```python
from build123d import *

# Parameters (mm, degrees)
F0_R             = 8
F1_DEPTH         = 1.5
F2_R             = 5.5
F3_DEPTH         = 22.5
F4_R             = 4
F5_DEPTH         = 21.5
F7_D             = 1.7
F9_D             = 3
F11_DEPTH        = 8.001
F11_DEPTH_BACK   = 25
F13_DEPTH        = 4
F13_COPIES_COUNT = 3


# Not quite as in the source:
# - a pattern or mirror of a feature is missing from the dataset's text; its kind, count and spacing are read off the source's solid


with BuildPart() as f1:
    # F0 (on Right) → F1 (new body)
    with BuildSketch(Plane.YZ):
        Circle(F0_R)
    extrude(amount=F1_DEPTH)

    # F2 (on face) → F3 (join)
    with BuildSketch(Plane.YZ.offset(1.5)):
        Circle(F2_R)
    extrude(amount=F3_DEPTH)

    # F4 (on face) → F5 (cut)
    with BuildSketch(Plane.YZ.offset(24)):
        Circle(F4_R)
    extrude(amount=-F5_DEPTH, mode=Mode.SUBTRACT)

    # F7 (through all)
    with Locations(Plane(origin=(0, 0, 0), x_dir=(0, 1, 0), z_dir=(-1, 0, 0))):
        with Locations((-3.25, -5.6291651246), (6.5, 0), (-3.25, 5.6291651246)):
            Hole(F7_D / 2)

    # F9 (through all)
    with Locations(Plane.YZ.offset(2.5)):
        with Locations((0, 0)):
            Hole(F9_D / 2)

    # F10 (on Front) → F11 (cut, two sides)
    with BuildSketch(Plane.XZ) as f11_sk:
        with BuildLine():
            Line((8, -1.75), (19.25, -1.75))
            ThreePointArc((19.25, -1.75), (21, 0), (19.25, 1.75))
            Line((19.25, 1.75), (8, 1.75))
            ThreePointArc((8, 1.75), (6.25, 0), (8, -1.75))
        make_face()
    extrude(amount=-F11_DEPTH, mode=Mode.SUBTRACT)
    extrude(f11_sk.sketch, amount=F11_DEPTH_BACK, mode=Mode.SUBTRACT)

    # F12 (on face) → F13 (cut)
    with BuildSketch(Plane.YZ.offset(1.5)):
        with BuildLine():
            Line((-0.5156865167, -5.4757709427), (-4.4843134833, -3.1844830952))
            ThreePointArc((-4.4843134833, -3.1844830952), (-3.702278018, -4.0673255927), (-2.7500001403, -4.7631396398))
            ThreePointArc((-2.7500001403, -4.7631396398), (-1.6712684341, -5.2399295626), (-0.5156865167, -5.4757709427))
        make_face()
    f13 = extrude(amount=F13_DEPTH, mode=Mode.SUBTRACT)

    # F13_copies: F13 ×3 about axis
    f13_copies_axis = Axis((0, 0, 0), (1, 0, 0))
    for i in range(1, F13_COPIES_COUNT):
        add(f13.rotate(f13_copies_axis, i * 360 / F13_COPIES_COUNT), mode=Mode.SUBTRACT)


solid = f1.part
```
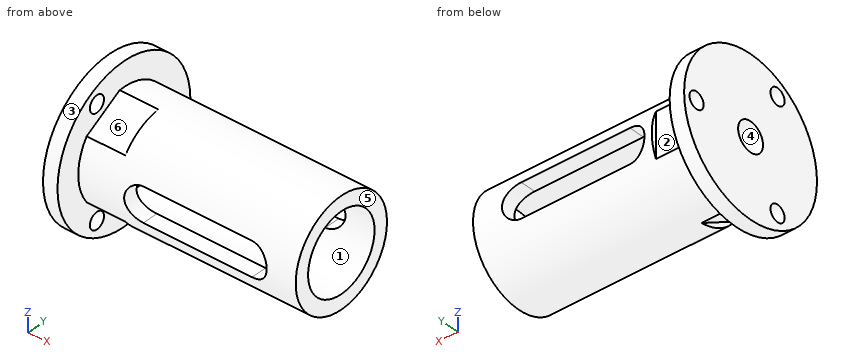
Design review of the part built by this model. Coordinates are the model's own, in mm. Face numbers are marked on the shaded views. A direction names the side the tool comes from. Give positions to 0.01 mm unless a question says otherwise; leave off trailing zeros. Loops run counter-clockwise (first coordinate to the right, second up) from the corner with the lowest first, then second, coordinate; pieces in that order, holes last. Notation, with made-up numbers: M 77.5,4.25 L 102.5,4.25 A17 cw 102.5,19.25 Z; hole C -13,-37.5 d11. An arc over 180 degrees is marked long. Return JSON: item names as keys, results as strings. Group by question number.
Item 1: For probe 1 along X at (y, z) = (-2.5, -4.5); probe 2 along Z at (x, y) = (10, 0); probe 3 along Z at (x, y) = (1.35, 0), list the stretches that pass through material, from the lowest coordinate up.
Item 2: We need section C-C (z = 0). Give the number of separate pieces and of enclosed holes in the cut face, and give its area (3 significant figures).
Item 3: We need section A-A (y = 0). Give the boundary of the cut face in (x, z).
Item 4: Tool access review of the marked faces 1, 2 and 3: name each direction out of +Z, -Z, +X, -X, +Y, -Y from which nothing blocks a thin tool from reaching the whole face with its end or side.
Item 5: We need section D-D (x = 3.25). Give the boundary of the cut face in (y, z).
Item 6: We need section B-B (x = 13.5). Give the boundary of the cut face in (y, z).
Item 7: Insertion check: pin 1 Ø3 at (x, z) = (11, -2) entering from +Y; pin 2 Ø6 at (x, z) = (8.5, 3) entering from +Y; pin 3 Ø0.5 at (x, y) = (15, 4.5) entering from +Z. Each pin has a flat end and moves straight along its axis. Give the tip position at first contact, or say it passes through.
Item 8: Mouldability with a two-part tool opening along X and no side actions: class the marked faces 4, 5 and 6 as released by +X, released by -X, zero draft, split by the parting line, or undercut.
Output:
{
 "1": {"probe 1": "x = 0 to 1.5, 5.5 to 24", "probe 2": "z = -5.5 to -4, 4 to 5.5", "probe 3": "z = -8 to -1.5, 1.5 to 8"},
 "2": {"separate pieces": "5", "enclosed holes": "0", "area": "43.2 mm^2"},
 "3": {"outline": "M 0,-8 L 1.5,-8 L 1.5,-5.5 L 24,-5.5 L 24,-4 L 2.5,-4 L 2.5,-1.5 L 0,-1.5 Z; M 0,1.5 L 2.5,1.5 L 2.5,4 L 24,4 L 24,5.5 L 1.5,5.5 L 1.5,8 L 0,8 Z"},
 "4": {"face 1": "+X", "face 2": "+Z, -Z, +Y", "face 3": "+X, -X"},
 "5": {"outline": "M -4.48,-3.18 L -0.52,-5.48 A5.5 ccw 5,-2.29 L 5,2.29 A5.5 ccw -0.52,5.48 L -4.48,3.18 A5.5 ccw Z; hole C 0,0 d8"},
 "6": {"outline": "M -5.21,-1.75 A5.5 ccw 5.21,-1.75 L 3.6,-1.75 A4 cw -3.6,-1.75 Z; M -5.21,1.75 L -3.6,1.75 A4 cw 3.6,1.75 L 5.21,1.75 A5.5 ccw Z"},
 "7": {"pin 1": "stops at y = 5.21", "pin 2": "stops at y = 5.44", "pin 3": "stops at z = 3.49"},
 "8": {"face 4": "zero draft", "face 5": "released by +X", "face 6": "undercut"}
}
